The figure shows three views and two pictorial views of one solid part (mm, origin at its lowest corner). Answer the questions. Round coordinates to 2 decimals unless told otherwise and drop trailing zeros. Order: outer loops, then holes, each group sorted by start corner. A loop starts at its lowest first (then second) coordinate and runs counter-clockwise, first axis right, second up. Notation, with made-up numbers: (9.25, 25.5) -> (41.25, 25.5) arc R19 ccw to (41.25, 42.5) -> close; hole circle Ø10 at (55.25, 85). An arc over 180 degrees is marked (long way). Return JSON: item names as keys, results as strings. Group by question number.
(1) The part is cut by section A-A (x = 17). Determine the outline of the cut face in (y, z) (1 decimal).
(2) The part is cut by section C-C (z = 1.3). Determine the outline of the cut face in (x, y) (1 decimal).
(3) This flat-tipped pin is pushed along its axis until it touches: pin 1 (1 mm diameter, centred on y = 32.5, z = 1.5, fed in from -X). Where does it stop, or does it pass through?
(4) The part is cut by section B-B (y = 40). Determine the outline of the cut face in (x, z) (1 decimal).
(5) Consider line 1 (X direction, y = 17, z = 2.2); line 2 (Y direction, x = 19.5, z = 2.3); line 3 (X direction, y = 76, z = 2.8). Determine where each line is inside the solid, lowest interval first. Write a range as [from, to].
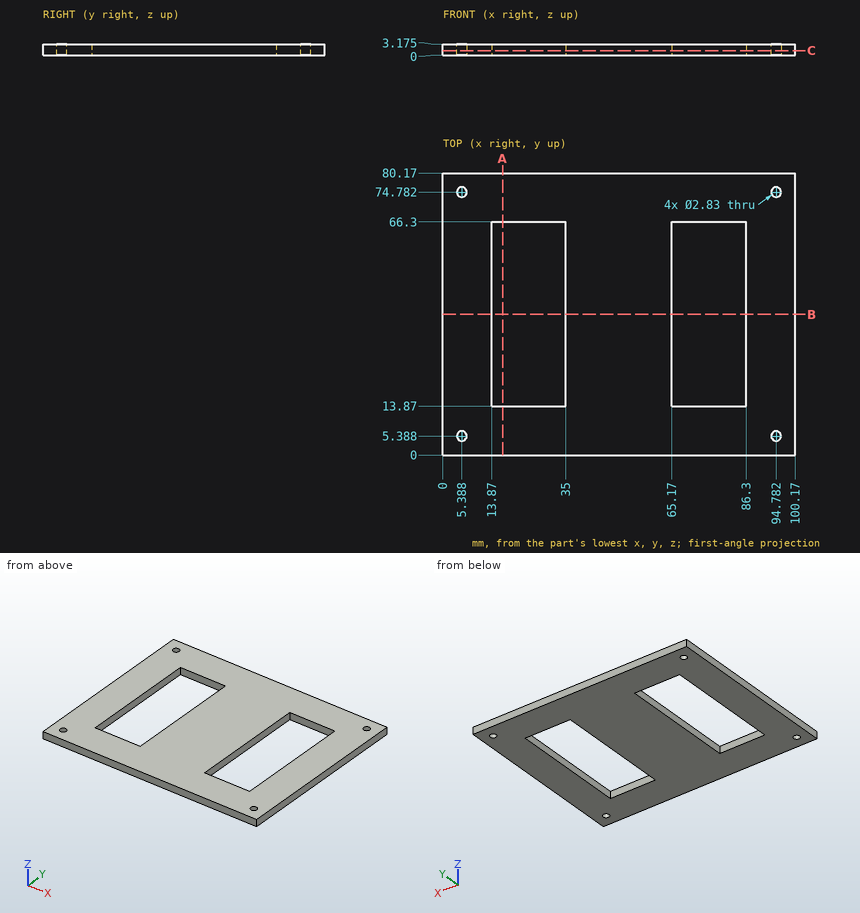
Answer below:
{
 "1": {"outline": "(0, 0) -> (13.9, 0) -> (13.9, 3.2) -> (0, 3.2) -> close; (66.3, 0) -> (80.2, 0) -> (80.2, 3.2) -> (66.3, 3.2) -> close"},
 "2": {"outline": "(0, 0) -> (100.2, 0) -> (100.2, 80.2) -> (0, 80.2) -> close; hole circle Ø2.8 at (5.4, 5.4); hole circle Ø2.8 at (5.4, 74.8); hole (13.9, 13.9) -> (35, 13.9) -> (35, 66.3) -> (13.9, 66.3) -> close; hole (65.2, 13.9) -> (86.3, 13.9) -> (86.3, 66.3) -> (65.2, 66.3) -> close; hole circle Ø2.8 at (94.8, 5.4); hole circle Ø2.8 at (94.8, 74.8)"},
 "3": {"pin 1": "stops at x = 0"},
 "4": {"outline": "(0, 0) -> (13.9, 0) -> (13.9, 3.2) -> (0, 3.2) -> close; (35, 0) -> (65.2, 0) -> (65.2, 3.2) -> (35, 3.2) -> close; (86.3, 0) -> (100.2, 0) -> (100.2, 3.2) -> (86.3, 3.2) -> close"},
 "5": {"line 1": "x = [0, 13.87], [35, 65.17], [86.3, 100.17]", "line 2": "y = [0, 13.87], [66.3, 80.17]", "line 3": "x = [0, 4.67], [6.11, 94.06], [95.5, 100.17]"}
}
